CAD build for the part. Positions are in the model's coordinates, mm. A direction names the side the tool comes from. Round coordinates to 2 decimals unless told otherwise and drop trailing zeros. Order: outer loops, then holes, each group sorted by start corner. A loop starts at its lowest first (then second) coordinate and runs counter-clockwise, first axis right, second up. Notation, with made-up numbers: M 0.5,30.25 L 51.5,30.25 A7 ccw 51.5,34.25 Z; hole C 25.25,69.25 d3. An arc over 180 degrees is marked long. Put each result on its own line as item: value.
```python
from build123d import *

# Parameters (mm, degrees)
SKETCH1_R           = 26.56205
BOSS_EXTRUDE2_DEPTH = 20
SKETCH2_W           = 20
SKETCH2_H           = 20
BOSS_EXTRUDE3_DEPTH = 40
SKETCH3_R           = 3.9773733
SKETCH3_R_2         = 3.985133
CUT_EXTRUDE1_DEPTH  = 159.491729693
FILLET1_R           = 5.08


with BuildPart() as part:
    # Sketch1 → Boss-Extrude2 (new body)
    # profile 1 of 3: a face of its own
    with BuildSketch(Plane(origin=(0, 0, 0), x_dir=(1, 0, 0), z_dir=(0, 1, 0))):
        with BuildLine():
            Line((37.922816996, -20), (37.922816996, 20))
            ThreePointArc((37.922816996, 20), (-42.873535531, 0), (37.922816996, -20))
        make_face()
        with Locations(Location((0, 0, 0), (0, 0, 270))):
            Circle(SKETCH1_R, mode=Mode.SUBTRACT)
    # profile 2 of 3: a face of its own
    with BuildSketch(Plane(origin=(0, 0, 0), x_dir=(1, 0, 0), z_dir=(0, 1, 0))):
        with BuildLine():
            Line((124.372816996, 20), (37.922816996, 20))
            ThreePointArc((37.922816996, 20), (41.617456018, 10.301815544), (42.873535531, 0))
            ThreePointArc((42.873535531, 0), (41.617456018, -10.301815544), (37.922816996, -20))
            Line((37.922816996, -20), (124.372816996, -20))
            Line((124.372816996, -20), (124.372816996, 20))
        make_face()
    # profile 3 of 3: a face of its own
    with BuildSketch(Plane(origin=(0, 0, 0), x_dir=(1, 0, 0), z_dir=(0, 1, 0))):
        with BuildLine():
            ThreePointArc((42.873535531, 0), (41.617456018, 10.301815544), (37.922816996, 20))
            Line((37.922816996, 20), (37.922816996, -20))
            ThreePointArc((37.922816996, -20), (41.617456018, -10.301815544), (42.873535531, 0))
        make_face()
    extrude(amount=BOSS_EXTRUDE2_DEPTH)

    # Sketch2 → Boss-Extrude3 (add)
    with BuildSketch(Plane(origin=(0, 0, -20), x_dir=(-1, 0, 0), z_dir=(0, 0, -1))):
        with Locations((-114.372816996, 30)):
            Rectangle(SKETCH2_W, SKETCH2_H)
    extrude(amount=-BOSS_EXTRUDE3_DEPTH)

    # Sketch3 → Cut-Extrude1 (cut, through all)
    with BuildSketch(Plane.ZY.offset(-104.372816996)):
        with Locations((9.96192, 31.22176)):
            Circle(SKETCH3_R)
        with Locations((-9.96192, 31.22176)):
            Circle(SKETCH3_R_2)
    extrude(amount=-CUT_EXTRUDE1_DEPTH, mode=Mode.SUBTRACT)

    # Fillet1
    fillet1_edges = [part.edges().sort_by_distance(p)[0] for p in [
        (104.372816996, 20, 0),
    ]]
    fillet(fillet1_edges, radius=FILLET1_R)


solid = part.part
```
Item 1: Band-saw the part on D-D on y = 33.5. Give the cut face in (x, z), and give its area (3 significant figures).
Answers below:
outline: M 104.37,-20 L 124.37,-20 L 124.37,-13.23 L 104.37,-13.23 Z; M 104.37,-6.69 L 124.37,-6.69 L 124.37,6.7 L 104.37,6.7 Z; M 104.37,13.22 L 124.37,13.22 L 124.37,20 L 104.37,20 Z
area: 539 mm²
Item 2: Band-saw the part on B-B on x = 0. Give the cut face in (y, z).
Answers below:
outline: M 0,-42.87 L 20,-42.87 L 20,-26.56 L 0,-26.56 Z; M 0,26.56 L 20,26.56 L 20,42.87 L 0,42.87 Z
Item 3: Mould opens along Z. For faces 1 (the flat face through (91, 16, 20)), 2 (the cylindrical face through (114.233, 33.915, -12.899)), 3 (the flat face through (115, 40, 0)), 4 (the cylindrical face through (114.233, 27.693, 11.797)) say: pulls with the +Z half, pulls with the -Z half, needs draft (parallel to the pull), parting line crosses it, or undercut.
Answers below:
face 1: pulls with the +Z half
face 2: undercut
face 3: needs draft
face 4: undercut
Item 4: Tool access for faces 5 (the flat face through (27, 20, -1)), 6 (the flat face through (91, 16, -20)), 7 (the flat face through (124.373, 20, 0)): list every direction of +Z, -Z, +X, -X, +Y, -Y with a clear straight run to the whole face (end or side of a thin tool).
Answers below:
face 5: +Z, -Z, -X, +Y
face 6: -Z, +X, +Y, -Y
face 7: +Z, -Z, +X, +Y, -Y
Item 5: Probe line 1 along X through (y, z) = (7, 0); line 2 along Y through (x, z) = (34.5, -20); line 3 along X through (y, z) = (25.5, 1.5). List the from-to ranges inside material, lowest first. Write a range as [from, to].
Answers below:
line 1: [-42.87, -26.56], [26.56, 124.37]
line 2: [0, 20]
line 3: [104.37, 124.37]
Item 6: Band-saw the part on A-A on z = 0. Give the cut face in (x, y), and give its area (3 significant figures).
Answers below:
outline: M -42.87,0 L -26.56,0 L -26.56,20 L -42.87,20 Z; M 26.56,0 L 124.37,0 L 124.37,40 L 104.37,40 L 104.37,25.08 A5.08 cw 99.29,20 L 26.56,20 Z
area: 2,690 mm²
Item 7: Pin check, flat tips, straight feed: P1, Ø2, axis at x = 76, z = -11, coming from the +Y side; P2, Ø7.5, axis at y = 31, z = 0.5, coming from the -X side; P3, Ø20, axis at x = 85.5, y = 27, coming from the -Z side. Stop position of each tip, or through.
Answers below:
P1: y = 20
P2: x = 104.37
P3: z = -20
Item 8: Band-saw the part on C-C on y = 15. Give the cut face in (x, z).
Answers below:
outline: M 37.92,-20 L 124.37,-20 L 124.37,20 L 37.92,20 A42.87 ccw long Z; hole C 0,0 d53.12
